Model file for the job. Use its own axes, mm. A direction names the side the tool comes from. Give positions to 0.01 mm unless a question says otherwise; leave off trailing zeros. Loops run counter-clockwise (first coordinate to the right, second up) from the corner with the lowest first, then second, coordinate; pieces in that order, holes last. Notation, with made-up numbers: M 24,-17 L 28,-17 A21 ccw 28,-3 Z; hole C -35,-25.75 d8. An arc over 180 degrees is marked long. Use CSV: the item, a comma, the result in double quotes. Start each with the question number.
(1) Slice it at A-A on z = -12.7. List the corners of the cut face in (x, y), and give its area (3 significant figures).
(2) Tool access for faces 5 (the face through (12, 19, 0)), 6 (the face through (-50, 38.1, -6)), 7 (the face through (0, 19, 18)), 8 (the face through (-50, 0, -6)): list every direction of +Z, -Z, +X, -X, +Y, -Y with a clear straight run to the whole face (end or side of a thin tool).
(3) Slice it at B-B on x = 12.7. List the corners of the cut face in (y, z).
(4) Wall check: line 1 along Y through (x, z) = (12.7, 9.75); line 2 along Y through (x, z) = (12, 11); line 3 along Z through (x, y) = (-26, 16) (3 decimals). Give the ranges that are in metal, low to high. Write a range as from..to.
(5) Two-plate mould, pull along X, no slides. Class faces 1 (the face through (6.09, -10.844, 10.181)), 2 (the face through (-35, 19, 15.875)), 3 (the face through (15.267, 33.165, 10.181)), 4 (the face through (-53.082, 18.783, -19.996)): pulls with the +X half, pulls with the -X half, needs draft (parallel to the pull), parting line crosses it, or undercut.
(6) Slice it at D-D on x = -8. List the corners of the cut face in (y, z) (3 decimals), and give its area (3 significant figures).
(7) Flat gauge pins, fed straight in: P1, Ø13, axis at x = 12.7, y = 0, coming from the -Z side; P2, Ø1.5, axis at x = -7, z = 7.5, coming from the +Y side; P3, Ø12, axis at y = 7, z = -22.5, coming from the -X side. Where does each tip first touch, or does it go through?
(8) Slice it at C-C on y = -4. List the corners of the cut face in (x, z).
```python
from build123d import *

# Parameters (mm, degrees)
F0_R     = 5.5626
F1_DEPTH = 20.6502
F2_R     = 19.05
F3_DEPTH = 38.1


with BuildPart() as f1:
    # F0 (on Top) → F1 (new body)
    with BuildSketch(Plane.XY):
        with BuildLine():
            Line((0, 38.1), (0, 0))
            ThreePointArc((0, 0), (6.247883, -10.93893), (18.844124, -11.114843))
            Line((18.844124, -11.114843), (52.188654, 7.317527))
            ThreePointArc((52.188654, 7.317527), (58.748963, 18.258285), (52.496517, 29.377852))
            Line((52.496517, 29.377852), (19.66947, 48.716802))
            ThreePointArc((19.66947, 48.716802), (6.667682, 49.275918), (0, 38.1))
        make_face()
        with Locations((12.7, 0)):
            Circle(F0_R, mode=Mode.SUBTRACT)
        with Locations((46.0502, 18.435503)):
            Circle(F0_R, mode=Mode.SUBTRACT)
        with Locations((12.7, 38.1)):
            Circle(F0_R, mode=Mode.SUBTRACT)
    extrude(amount=F1_DEPTH)

    # F2 (on Front) → F3 (join)
    with BuildSketch(Plane.XZ):
        with BuildLine():
            Line((0, 0), (0, 15.875))
            Line((0, 15.875), (-70.678988, 15.875))
            ThreePointArc((-70.678988, 15.875), (-81.204468, 13.86586), (-90.249832, 8.120968))
            ThreePointArc((-90.249832, 8.120968), (-79.38338, -39.916983), (-42.658184, -7.099542))
            ThreePointArc((-42.658184, -7.099542), (-39.261941, -1.980859), (-33.44717, 0))
            Line((-33.44717, 0), (0, 0))
        make_face()
        with Locations((-70.678988, -12.7)):
            Circle(F2_R, mode=Mode.SUBTRACT)
    extrude(amount=-F3_DEPTH)


solid = f1.part
```
Reply:
1,outline,"M -99.25,0 L -89.73,0 L -89.73,38.1 L -99.25,38.1 Z; M -51.63,0 L -42.1,0 L -42.1,38.1 L -51.63,38.1 Z"
1,area,"726 mm^2"
2,face 5,"-Z, +X, +Y, -Y"
2,face 6,"+Z, -Z, -X, +Y"
2,face 7,"+Z, -X, +Y, -Y"
2,face 8,"+Z, -Z, -X, -Y"
3,outline,"M -12.7,0 L -5.56,0 L -5.56,20.65 L -12.7,20.65 Z; M 5.56,0 L 32.54,0 L 32.54,20.65 L 5.56,20.65 Z; M 43.66,0 L 50.8,0 L 50.8,20.65 L 43.66,20.65 Z"
4,line 1,"y = -12.7..-5.56, 5.56..32.54, 43.66..50.8"
4,line 2,"y = -12.68..-5.52, 5.52..32.58, 43.62..50.78"
4,line 3,"z = 0..15.875"
5,face 1,"parting line crosses it"
5,face 2,"needs draft"
5,face 3,"undercut"
5,face 4,"undercut"
6,outline,"M 0,0 L 38.1,0 L 38.1,15.875 L 0,15.875 Z"
6,area,"605 mm^2"
7,P1,"stops at z = 0"
7,P2,"stops at y = 38.1"
7,P3,"stops at x = -99"
8,outline,"M 0.65,0 L 8.83,0 L 8.83,20.65 L 0.65,20.65 Z; M 16.57,0 L 31.72,0 L 31.72,20.65 L 16.57,20.65 Z"
